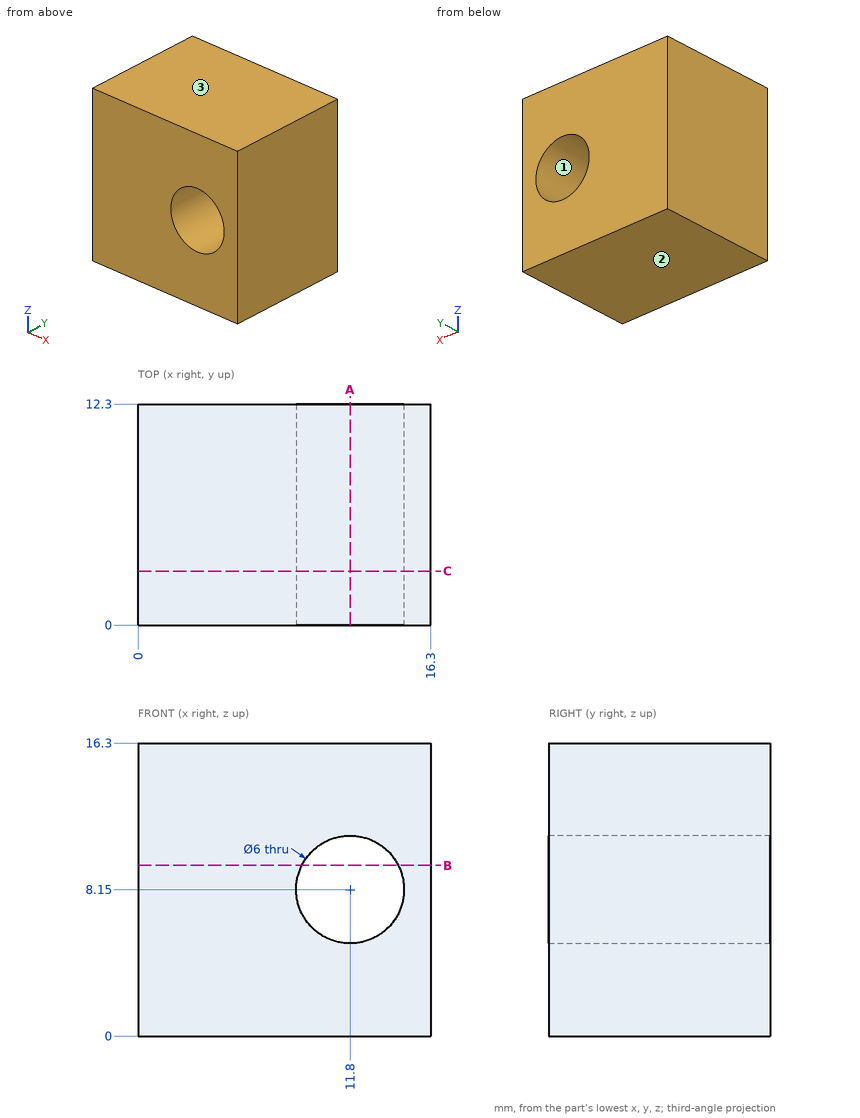
Geometry: see drawing. Coordinates: mm, zero at the bounding-box minimum. Coordinates: 2 decimals unless noted, no trailing zeros. Loops run counter-clockwise (first coordinate to the right, second up) from the corner with the lowest first, then second, coordinate; pieces in that order, holes last.
Q1. Cut plane A-A (x = 11.8). Output: boundary loops of the cut face in (y, z).
Q2. Draft query along Z for the marked faces 1, 2 and 3. Return one class per face: +Z half, -Z half, draft (parallel to the pull), parting line (faces both ways), or undercut.
Q3. Cut plane B-B (z = 9.5). Output: boundary loops of the cut face in (x, y).
Q4. Cut plane C-C (y = 3). Output: boundary loops of the cut face in (x, z), then the cut area to 3 significant figures.
Q5. Material intervals for line 1 (Z direction, x = 11.8, y = 6); line 2 (X direction, y = 3, z = 8.15); line 3 (Z direction, x = 10, y = 4.75), sorted ascending.
Q6. Contact query for a flat-ended pin moving along its axis: pin 1 (1.5 mm diameter, centred on y = 8.5, z = 3.5, fed in from -X). Output: stop coordinate, or through.
Working result:
1. outline: (0, 0) - (12.3, 0) - (12.3, 5.15) - (0, 5.15) - close; (0, 11.15) - (12.3, 11.15) - (12.3, 16.3) - (0, 16.3) - close
2. face 1: undercut
2. face 2: -Z half
2. face 3: +Z half
3. outline: (0, 0) - (9.12, 0) - (9.12, 12.3) - (0, 12.3) - close; (14.48, 0) - (16.3, 0) - (16.3, 12.3) - (14.48, 12.3) - close
4. outline: (0, 0) - (16.3, 0) - (16.3, 16.3) - (0, 16.3) - close; hole circle Ø6 at (11.8, 8.15)
4. area: 237 mm2
5. line 1: z = 0 to 5.15, 11.15 to 16.3
5. line 2: x = 0 to 8.8, 14.8 to 16.3
5. line 3: z = 0 to 5.75, 10.55 to 16.3
6. pin 1: stops at x = 0
